from build123d import *

# Parameters (mm, degrees)
BOSS_EXTRUDE1_DEPTH = 10
SKETCH2_R           = 2.5
CUT_EXTRUDE1_DEPTH  = 21
SKETCH3_R           = 6
CUT_EXTRUDE2_DEPTH  = 5
SKETCH4_R           = 5.2
BOSS_EXTRUDE2_DEPTH = 5


with BuildPart() as part:
    # Sketch1 → Boss-Extrude1 (new body)
    with BuildSketch(Plane(origin=(0, 0, 0), x_dir=(1, 0, 0), z_dir=(0, 1, 0))):
        with BuildLine():
            Line((10.5, 19), (5.5, 19))
            Line((5.5, 19), (0.5, 19))
            Line((0.5, 19), (0.5, 14))
            Line((0.5, 14), (0.5, 4))
            Line((0.5, 4), (0.5, 3.968626967))
            ThreePointArc((0.5, 3.968626967), (3, 2.645751311), (4, 0))
            ThreePointArc((4, 0), (-2.645751311, -3), (-0.5, 3.968626967))
            Line((-0.5, 3.968626967), (-0.5, 4))
            Line((-0.5, 4), (-0.5, 14))
            Line((-0.5, 14), (-0.5, 19))
            Line((-0.5, 19), (-5.5, 19))
            Line((-5.5, 19), (-10.5, 19))
            Line((-10.5, 19), (-10.5, 10))
            Line((-10.5, 10), (-33, 10))
            Line((-33, 10), (-33, -10))
            Line((-33, -10), (-24, -10))
            Line((-24, -10), (24, -10))
            Line((24, -10), (33, -10))
            Line((33, -10), (33, 10))
            Line((33, 10), (10.5, 10))
            Line((10.5, 10), (10.5, 19))
        make_face()
    extrude(amount=BOSS_EXTRUDE1_DEPTH)

    # Sketch2 → Cut-Extrude1 (cut)
    with BuildSketch(Plane(origin=(10.5, 0, 0), x_dir=(0, 0, -1), z_dir=(1, 0, 0))):
        with Locations((14.5, 5)):
            Circle(SKETCH2_R)
    extrude(amount=-CUT_EXTRUDE1_DEPTH, mode=Mode.SUBTRACT)

    # Sketch3 → Cut-Extrude2 (cut)
    with BuildSketch(Plane(origin=(0, 10, 0), x_dir=(1, 0, 0), z_dir=(0, 1, 0))):
        with Locations(Location((24, 0, 0), (0, 0, 270))):
            Circle(SKETCH3_R)
        with Locations(Location((-24, 0, 0), (0, 0, 270))):
            Circle(SKETCH3_R)
    extrude(amount=-CUT_EXTRUDE2_DEPTH, mode=Mode.SUBTRACT)

    # Sketch4 → Boss-Extrude2 (add)
    with BuildSketch(Plane(origin=(0, 5, 0), x_dir=(1, 0, 0), z_dir=(0, 1, 0))):
        with Locations(Location((24, 0, 0), (0, 0, 270))):
            Circle(SKETCH4_R)
        with Locations(Location((-24, 0, 0), (0, 0, 270))):
            Circle(SKETCH4_R)
    extrude(amount=BOSS_EXTRUDE2_DEPTH)


solid = part.part
Model file for the job. Use its own axes, mm. A direction names the side the tool comes from. Give positions to 0.01 mm unless a question says otherwise; leave off trailing zeros. Order: outer loops, then holes, each group sorted by start corner. A loop starts at its lowest first (then second) coordinate and runs counter-clockwise, first axis right, second up. Notation, with made-up numbers: M 17,52.5 L 31,52.5 A19 ccw 31,62.5 Z; hole C 29,22 d2. An arc over 180 degrees is marked long. Put each result on its own line as item: value. Start each with the question number.
(1) Band-saw the part on A-A on y = 8.5. Give the cut face in (x, z).
(2) Pin check, flat tips, straight feed: pin 1 Ø4.5 at (y, z) = (4.5, -12.5) entering from -X; pin 2 Ø8 at (x, z) = (-23.5, -12) entering from -Y; pin 3 Ø3 at (x, y) = (-21.5, 5.5) entering from -Z. Stop position of each tip, or through.
(3) Drill centre lines: L1, parallel to X at y = 8.6, z = 0; L2, parallel to X at y = 4.5, z = 0; L3, parallel to X at y = 2.75, z = -13. Where is each one in solid material? Low to high. Write a range as [from, to].
(4) Tool access for faces 4 (the face through (-10.5, 3, -17)), 5 (the face through (-29.076, 7.465, -1.127)), 6 (the face through (0.5, 4.9, -11.6)), 7 (the face through (33, 5, 0)), 8 (the face through (0, 10, 5)): list every direction of +Z, -Z, +X, -X, +Y, -Y with a clear straight run to the whole face (end or side of a thin tool).
(5) Band-saw the part on B-B on z = -14.5. Give the cut face in (x, y), then the cut area to 3 significant figures.
(6) Pull direction Z, two halves, no side cores. Call faces 1 (the face through (-0.5, 5, -11)), 2 (the face through (-5, 5, -12)), 3 (the face through (22, 5, -10)): released by +Z, released by -Z, zero draft, split by the parting line, or undercut.
(7) Band-saw the part on D-D on x = -24. Give the cut face in (y, z), then the cut area to 3 significant figures.
(8) Band-saw the part on C-C on z = 1.25. Give the cut face in (x, y).
Results below:
1. outline: M -33,-10 L -10.5,-10 L -10.5,-19 L -0.5,-19 L -0.5,-3.97 A4 cw long 0.5,-3.97 L 0.5,-19 L 10.5,-19 L 10.5,-10 L 33,-10 L 33,10 L -33,10 Z; C -24,0 d10.4; C 24,0 d10.4; hole C -24,0 d12; hole C 24,0 d12
2. pin 1: stops at x = -10.5
2. pin 2: stops at y = 0
2. pin 3: stops at z = -10
3. L1: x = [-33, -30], [-29.2, -18.8], [-18, -4], [4, 18], [18.8, 29.2], [30, 33]
3. L2: x = [-33, -4], [4, 33]
3. L3: x = [-10.5, -0.5], [0.5, 10.5]
4. face 4: -Z, -X, +Y, -Y
4. face 5: +Y
4. face 6: -Z, +Y, -Y
4. face 7: +Z, -Z, +X, +Y, -Y
4. face 8: +Z, -Z, +X, -X, +Y
5. outline: M -10.5,0 L -0.5,0 L -0.5,2.5 L -10.5,2.5 Z; M -10.5,7.5 L -0.5,7.5 L -0.5,10 L -10.5,10 Z; M 0.5,0 L 10.5,0 L 10.5,2.5 L 0.5,2.5 Z; M 0.5,7.5 L 10.5,7.5 L 10.5,10 L 0.5,10 Z
5. area: 100 mm2
6. face 1: zero draft
6. face 2: undercut
6. face 3: released by -Z
7. outline: M 0,-10 L 10,-10 L 10,-6 L 5,-6 L 5,-5.2 L 10,-5.2 L 10,5.2 L 5,5.2 L 5,6 L 10,6 L 10,10 L 0,10 Z
7. area: 192 mm2
8. outline: M -33,0 L -3.8,0 L -3.8,10 L -18.13,10 L -18.13,5 L -18.95,5 L -18.95,10 L -29.05,10 L -29.05,5 L -29.87,5 L -29.87,10 L -33,10 Z; M 3.8,0 L 33,0 L 33,10 L 29.87,10 L 29.87,5 L 29.05,5 L 29.05,10 L 18.95,10 L 18.95,5 L 18.13,5 L 18.13,10 L 3.8,10 Z
